from build123d import *

# Parameters (mm, degrees)
SKETCH1_R            = 50.8
BOSS_EXTRUDE3_DEPTH  = 50.8
SKETCH5_R            = 7.62
CUT_EXTRUDE2_DEPTH   = 50.8
SKETCH6_W            = 101.31384703
SKETCH6_H            = 7.62
SKETCH6_W_2          = 7.62
SKETCH6_H_2          = 101.31384703
BOSS_EXTRUDE4_DEPTH  = 7.62
SKETCH7_R            = 5.08
BOSS_EXTRUDE5_DEPTH  = 1.27
SKETCH8_R            = 2.54
BOSS_EXTRUDE6_DEPTH  = 1.27
SKETCH9_R            = 2.54
BOSS_EXTRUDE7_DEPTH  = 76.2
SKETCH10_R           = 6.35
BOSS_EXTRUDE8_DEPTH  = 50.8
SKETCH11_W           = 7.62
SKETCH11_H           = 104.14
SKETCH11_W_2         = 104.14
SKETCH11_H_2         = 7.62
BOSS_EXTRUDE9_DEPTH  = 7.62
SKETCH12_R           = 6.35
BOSS_EXTRUDE10_DEPTH = 1.27


with BuildPart() as part:
    # Sketch1 → Boss-Extrude3 (new body)
    with BuildSketch(Plane.XY):
        Circle(SKETCH1_R)
    extrude(amount=BOSS_EXTRUDE3_DEPTH)

    # Sketch5 → Cut-Extrude2 (cut)
    with BuildSketch(Plane.XY.offset(50.8)):
        with Locations((0, 14.676826076)):
            Circle(SKETCH5_R)
        with Locations((7.338413038, 12.710504229)):
            Circle(SKETCH5_R)
        with Locations((12.710504229, 7.338413038)):
            Circle(SKETCH5_R)
        with Locations((14.676826076, 0)):
            Circle(SKETCH5_R)
        with Locations((12.710504229, -7.338413038)):
            Circle(SKETCH5_R)
        with Locations((7.338413038, -12.710504229)):
            Circle(SKETCH5_R)
        with Locations((0, -14.676826076)):
            Circle(SKETCH5_R)
        with Locations((-7.338413038, -12.710504229)):
            Circle(SKETCH5_R)
        with Locations((-12.710504229, -7.338413038)):
            Circle(SKETCH5_R)
        with Locations((-14.676826076, 0)):
            Circle(SKETCH5_R)
        with Locations((-12.710504229, 7.338413038)):
            Circle(SKETCH5_R)
        with Locations((-7.338413038, 12.710504229)):
            Circle(SKETCH5_R)
    extrude(amount=-CUT_EXTRUDE2_DEPTH, mode=Mode.SUBTRACT)


with BuildPart() as cut_extrude2_piece_1:
    # of the separate pieces the step leaves, piece 1, a body of its own (cut_extrude2_pieces)
    add(part.part.solids().sort_by_distance((50.8, 0, 0))[0])



with BuildPart() as cut_extrude2_piece_2:
    # of the separate pieces the step leaves, piece 2, a body of its own (cut_extrude2_pieces)
    add(part.part.solids().sort_by_distance((-5.35355304, 5.35355304, 0))[0])


with BuildPart() as cut_extrude2_piece_1_1:
    add(cut_extrude2_piece_1.part)

    add(cut_extrude2_piece_2.part)  # Boss-Extrude4 merges Cut-Extrude2 piece 2
    # Sketch6 → Boss-Extrude4 (add)
    with BuildSketch(Plane.XY.offset(50.8)):
        Rectangle(SKETCH6_W, SKETCH6_H)
        Rectangle(SKETCH6_W_2, SKETCH6_H_2)
    extrude(amount=-BOSS_EXTRUDE4_DEPTH)

    # Sketch7 → Boss-Extrude5 (add)
    with BuildSketch(Plane.XY.offset(50.8)):
        Circle(SKETCH7_R)
    extrude(amount=BOSS_EXTRUDE5_DEPTH)

    # Sketch8 → Boss-Extrude6 (add)
    with BuildSketch(Plane.XY.offset(52.07)):
        Circle(SKETCH8_R)
    extrude(amount=BOSS_EXTRUDE6_DEPTH)

    # Sketch9 → Boss-Extrude7 (add)
    with BuildSketch(Plane(origin=(0, 0, 0), x_dir=(-1, 0, 0), z_dir=(0, 0, -1))):
        with Locations(Location((0, 0, 0), (0, 0, 180))):
            Circle(SKETCH9_R)
    extrude(amount=BOSS_EXTRUDE7_DEPTH)

    # Sketch10 → Boss-Extrude8 (add)
    with BuildSketch(Plane.XY.offset(50.8)):
        with Locations((0, 46.99)):
            Circle(SKETCH10_R)
        with Locations((12.161906929, 45.388854577)):
            Circle(SKETCH10_R)
        with Locations((23.495, 40.694533724)):
            Circle(SKETCH10_R)
        with Locations((33.226947648, 33.226947648)):
            Circle(SKETCH10_R)
        with Locations((40.694533724, 23.495)):
            Circle(SKETCH10_R)
        with Locations((45.388854577, 12.161906929)):
            Circle(SKETCH10_R)
        with Locations((46.99, 0)):
            Circle(SKETCH10_R)
        with Locations((45.388854577, -12.161906929)):
            Circle(SKETCH10_R)
        with Locations((40.694533724, -23.495)):
            Circle(SKETCH10_R)
        with Locations((33.226947648, -33.226947648)):
            Circle(SKETCH10_R)
        with Locations((23.495, -40.694533724)):
            Circle(SKETCH10_R)
        with Locations((12.161906929, -45.388854577)):
            Circle(SKETCH10_R)
        with Locations((0, -46.99)):
            Circle(SKETCH10_R)
        with Locations((-12.161906929, -45.388854577)):
            Circle(SKETCH10_R)
        with Locations((-23.495, -40.694533724)):
            Circle(SKETCH10_R)
        with Locations((-33.226947648, -33.226947648)):
            Circle(SKETCH10_R)
        with Locations((-40.694533724, -23.495)):
            Circle(SKETCH10_R)
        with Locations((-45.388854577, -12.161906929)):
            Circle(SKETCH10_R)
        with Locations((-46.99, 0)):
            Circle(SKETCH10_R)
        with Locations((-45.388854577, 12.161906929)):
            Circle(SKETCH10_R)
        with Locations((-40.694533724, 23.495)):
            Circle(SKETCH10_R)
        with Locations((-33.226947648, 33.226947648)):
            Circle(SKETCH10_R)
        with Locations((-23.495, 40.694533724)):
            Circle(SKETCH10_R)
        with Locations((-12.161906929, 45.388854577)):
            Circle(SKETCH10_R)
    extrude(amount=-BOSS_EXTRUDE8_DEPTH)

    # Sketch11 → Boss-Extrude9 (add)
    with BuildSketch(Plane(origin=(0, 0, 0), x_dir=(-1, 0, 0), z_dir=(0, 0, -1))):
        Rectangle(SKETCH11_W, SKETCH11_H)
        Rectangle(SKETCH11_W_2, SKETCH11_H_2)
    extrude(amount=-BOSS_EXTRUDE9_DEPTH)

    # Sketch12 → Boss-Extrude10 (add)
    with BuildSketch(Plane(origin=(0, 0, 0), x_dir=(-1, 0, 0), z_dir=(0, 0, -1))):
        with Locations(Location((0, 0, 0), (0, 0, 180))):
            Circle(SKETCH12_R)
    extrude(amount=BOSS_EXTRUDE10_DEPTH)


solid = cut_extrude2_piece_1_1.part
Check sheet for the modelled part. Datum: model origin and axes. Units: mm. A direction names the side the tool comes from. Give positions to 0.01 mm unless a question says otherwise; leave off trailing zeros. Order: outer loops, then holes, each group sorted by start corner. A loop starts at its lowest first (then second) coordinate and runs counter-clockwise, first axis right, second up. Notation, with made-up numbers: M 19.5,-14 L 33.5,-14 A14 cw 33.5,5 Z; hole C 5.5,88 d6. An arc over 180 degrees is marked long. Answer as CSV lines item,"result". Start each with the question number.
Item 1: Mould release check, pull along Y, two halves, no side actions. Record for faces 6 (the face through (-0.33, -2.52, -38.21)), 7 (the face through (-14, 0, 43.18)), 8 (the face through (-19.27, 11.22, 25.76)), 9 (the face through (2, -2, 52.07)): +Y half, -Y half, draft (parallel to the pull), parting line (faces both ways), or undercut.
Item 2: Gauge pin test, flat ends, axial feed: P1, Ø8, axis at x = 18, z = 19.5, coming from the +Y side; P2, Ø12, axis at y = -24.5, z = 19, coming from the +X side; P3, Ø8, axis at x = -5, y = -5, coming from the +Z side. Record the tip position at first contact, or that the pin passes through.
Item 3: Thickness scan on line 1 (Y direction, x = 6.5, z = 23); line 2 (Z direction, x = 32, y = 24.5); line 3 (Y direction, x = -5, z = 22). Record the ranges inside material, lowest first. Write a range as [from, to].
Item 4: Cross-section at C-C on y = 11.5. Enter the section's corners in (x, z), plus the area to 3 significant figures.
Item 5: Cross-section at D-D on z = -8.5. Enter the section's corners in (x, y).
Item 6: Tool access check on faces 1 (the face through (-14, 3.81, 47)), 2 (the face through (0.028, -7.057, 25.649)), 3 (the face through (-0.33, 2.52, 52.7)), 4 (the face through (-13.721, 51.544, 25.756)), 5 (the face through (26.59, -46.24, 25.76)). Record the directions out of +Z, -Z, +X, -X, +Y, -Y that give a thin tool (end or side, any length) a straight path to the whole face; none if there is none.
Item 7: Cross-section at A-A on x = 0. Enter the section's corners in (y, z), plus the area to 3 significant figures.
Established:
1,face 6,"parting line"
1,face 7,"undercut"
1,face 8,"undercut"
1,face 9,"draft"
2,P1,"stops at y = 51.47"
2,P2,"stops at x = 47.31"
2,P3,"stops at z = 52.07"
3,line 1,"y = [-50.38, -20.28], [-2.92, 2.92], [20.28, 50.38]"
3,line 2,"z = [0, 50.8]"
3,line 3,"y = [-50.9, -20.43], [-5.46, 5.46], [20.43, 50.9]"
4,outline,"M -51.7,0 L -19.09,0 L -19.09,50.8 L -51.7,50.8 Z; M -3.81,0 L 3.81,0 L 3.81,7.62 L -3.81,7.62 Z; M -3.81,43.18 L 3.81,43.18 L 3.81,50.8 L -3.81,50.8 Z; M 19.09,0 L 51.7,0 L 51.7,50.8 L 19.09,50.8 Z"
4,area,"3,430 mm^2"
5,outline,"C 0,0 d5.08"
6,face 1,"+Z, -Z"
6,face 2,"none"
6,face 3,"+Z"
6,face 4,"+Z, -Z, +Y"
6,face 5,"+Z, -Z, -Y"
7,outline,"M -53.34,0 L -6.35,0 L -6.35,-1.27 L -2.54,-1.27 L -2.54,-76.2 L 2.54,-76.2 L 2.54,-1.27 L 6.35,-1.27 L 6.35,0 L 53.34,0 L 53.34,50.8 L 5.08,50.8 L 5.08,52.07 L 2.54,52.07 L 2.54,53.34 L -2.54,53.34 L -2.54,52.07 L -5.08,52.07 L -5.08,50.8 L -53.34,50.8 Z; hole M -22.3,7.62 L -7.06,7.62 L -7.06,43.18 L -22.3,43.18 Z; hole M 7.06,7.62 L 22.3,7.62 L 22.3,43.18 L 7.06,43.18 Z"
7,area,"4,750 mm^2"
